Geometry: see drawing. Coordinates: mm, zero at the bounding-box minimum. Round coordinates to 2 decimals unless told otherwise and drop trailing zeros. Order: outer loops, then holes, each group sorted by start corner. A loop starts at its lowest first (then second) coordinate and runs counter-clockwise, first axis right, second up. Notation, with made-up numbers: (-34.5, 54.5) -> (-11.5, 54.5) arc R33 cw to (-11.5, 88.5) -> close; hole circle Ø5 at (59.5, 67.25). An arc over 180 degrees is marked (long way). Put each result on its own line as item: value.
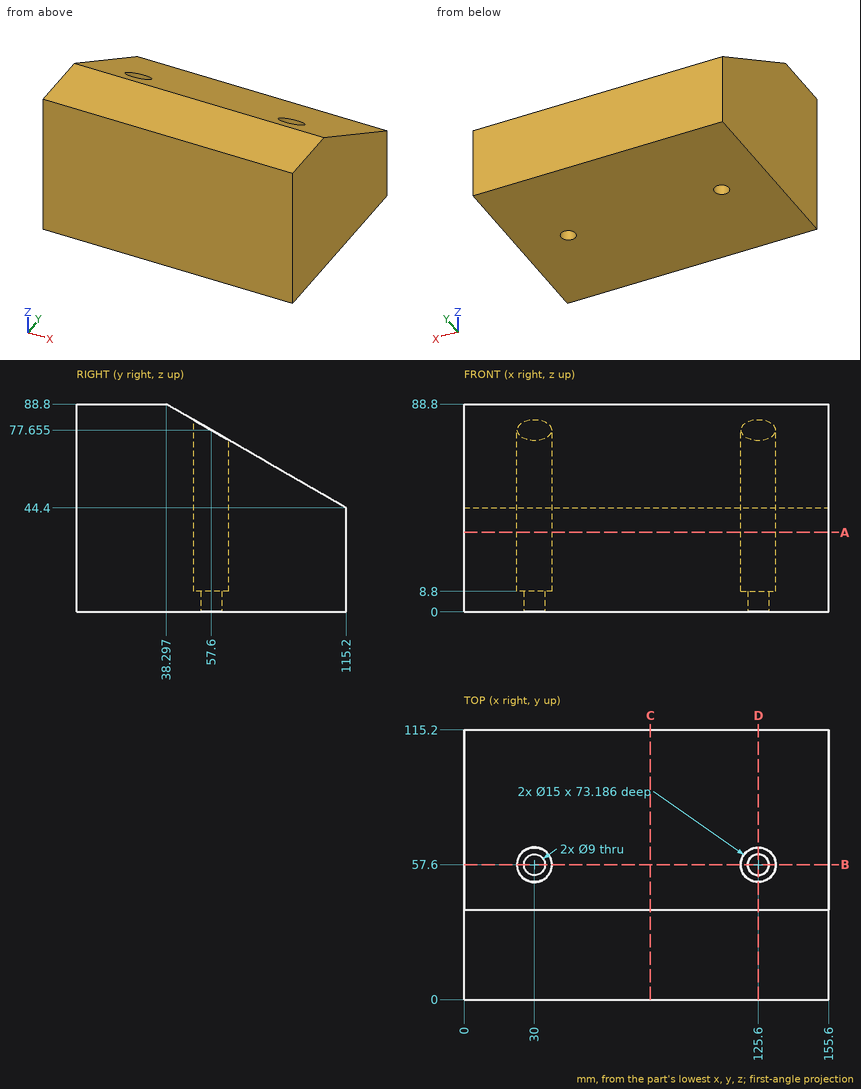
1. Cut plane B-B on y = 57.6. Return loops of the section in (x, z) (1 decimal), and give its area (3 significant figures).
Ans:
outline: (0, 0) -> (25.5, 0) -> (25.5, 8.8) -> (22.5, 8.8) -> (22.5, 77.7) -> (0, 77.7) -> close; (34.5, 0) -> (121.1, 0) -> (121.1, 8.8) -> (118.1, 8.8) -> (118.1, 77.7) -> (37.5, 77.7) -> (37.5, 8.8) -> (34.5, 8.8) -> close; (130.1, 0) -> (155.6, 0) -> (155.6, 77.7) -> (133.1, 77.7) -> (133.1, 8.8) -> (130.1, 8.8) -> close
area: 9,860 mm²
2. Cut plane C-C on x = 79.5. Return loops of the section in (y, z).
Ans:
outline: (0, 0) -> (115.2, 0) -> (115.2, 44.4) -> (38.3, 88.8) -> (0, 88.8) -> close
3. Contact query for flat-ended pins moving along their axis: P1, Ø7.5, axis at x = 30.5, y = 55, coming from the +Z side; P2, Ø8, axis at x = 30, y = 57.6, coming from the +Z side; P3, Ø1.5, axis at x = 66, z = 76, coming from the +Y side (1 decimal); P4, Ø17, axis at x = 125.6, y = 57.6, coming from the +Z side. Output: stop coordinate, or through.
Ans:
P1: z = 8.8
P2: through
P3: y = 61.8
P4: z = 82.56
4. Cut plane D-D on x = 125.6. Return loops of the section in (y, z) (1 decimal), and give its area (3 significant figures).
Ans:
outline: (0, 0) -> (53.1, 0) -> (53.1, 8.8) -> (50.1, 8.8) -> (50.1, 82) -> (38.3, 88.8) -> (0, 88.8) -> close; (62.1, 0) -> (115.2, 0) -> (115.2, 44.4) -> (65.1, 73.3) -> (65.1, 8.8) -> (62.1, 8.8) -> close
area: 7,410 mm²
5. Material intervals for probe 1 along Y at (x, z) = (30, 5); probe 2 along Y at (x, z) = (120.5, 47) (1 decimal); probe 3 along Z at (x, y) = (52.5, 51.5), sorted ascending.
Ans:
probe 1: 0 to 53.1, 62.1 to 115.2
probe 2: 0 to 52.1, 63.1 to 110.7
probe 3: 0 to 81.18
6. Cut plane A-A on z = 34. Return loops of the section in (x, y), and give its area (3 significant figures).
Ans:
outline: (0, 0) -> (155.6, 0) -> (155.6, 115.2) -> (0, 115.2) -> close; hole circle Ø15 at (30, 57.6); hole circle Ø15 at (125.6, 57.6)
area: 17,600 mm²
